Geometry check sheet. Reference: the model listing, model coordinates, mm. Face numbers are marked on the shaded views. A direction names the side the tool comes from. Coordinates: 2 decimals unless noted, no trailing zeros. Loops run counter-clockwise (first coordinate to the right, second up) from the corner with the lowest first, then second, coordinate; pieces in that order, holes last.
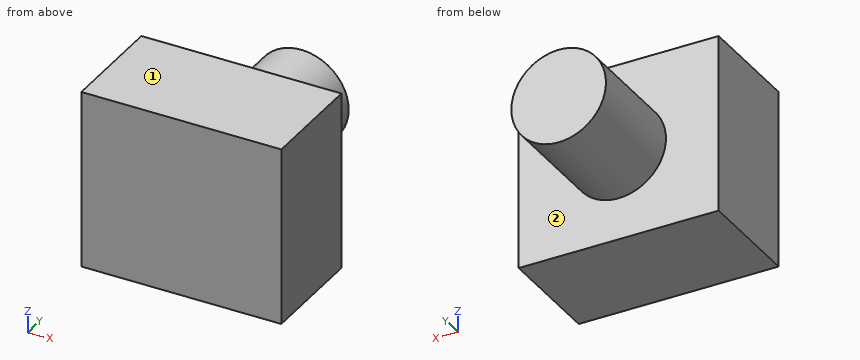
Autodesk Inventor part; units mm, degrees
ref_plane "YZ Plane" through (0, 0, 0) normal (1, 0, 0) x (0, 1, 0)
ref_plane "XZ Plane" through (0, 0, 0) normal (0, 1, 0) x (-1, 0, 0)
ref_plane "XY Plane" through (0, 0, 0) normal (0, 0, 1) x (1, 0, 0)
sketch "Эскиз1" plane through (0, 0, 0) normal (0, 1, 0) x (-1, 0, 0)
  line L0 (3.7, 3.3) -> (-3.7, 3.3)
  line L1 (-3.7, 3.3) -> (-3.7, -3.3)
  line L2 (-3.7, -3.3) -> (3.7, -3.3)
  line L3 (3.7, -3.3) -> (3.7, 3.3)
  point P0 (0, 0)
  dimension "d1" = 6.6
  dimension "d2" = 7.4
  dimension "d3" = 3.3
  dimension "d4" = 3.7
extrude "Выдавливание1" add sketch "Эскиз1" along normal blind 4
sketch "Эскиз2" plane through (0, 4, 0) normal (0, 1, 0) x (1, 0, 0)
  circle A0 centre (0, 0) radius 1.75
  dimension "d7" = 3.5
extrude "Выдавливание2" add sketch "Эскиз2" along normal blind 4
properties part number "btn"
(1) Sectioned sample at C-C on y = 5. Record the cut outline in (x, z), and give its area (3 significant figures).
Findings:
outline: circle Ø3.5 at (0, 0)
area: 9.62 mm2
(2) Access from +Z, -Z, +X, -X, +Y, -Y to the whole of each face (thin tool, end or side, straight path). Record for the marked faces 1 and 2.
Findings:
face 1: +Z, +X, -X, +Y, -Y
face 2: +Y
(3) Sectioned sample at A-A on x = 0. Record the cut outline in (y, z).
Findings:
outline: (0, -3.3) - (4, -3.3) - (4, -1.75) - (8, -1.75) - (8, 1.75) - (4, 1.75) - (4, 3.3) - (0, 3.3) - close
(4) Sectioned sample at D-D on z = -2. Record the cut outline in (x, y).
Findings:
outline: (-3.7, 0) - (3.7, 0) - (3.7, 4) - (-3.7, 4) - close
(5) Sectioned sample at B-B on z = 0. Record the cut outline in (x, y).
Findings:
outline: (-3.7, 0) - (3.7, 0) - (3.7, 4) - (1.75, 4) - (1.75, 8) - (-1.75, 8) - (-1.75, 4) - (-3.7, 4) - close
(6) Gauge pin test, flat ends, axial feed: pin 1 Ø1.5 at (y, z) = (5.5, 0) entering from +X; pin 2 Ø4 at (x, y) = (-2, 7) entering from -Z. Record the tip position at first contact, or that the pin passes through.
Findings:
pin 1: stops at x = 1.75
pin 2: stops at z = -1.75
(7) Scan lines: L1, parallel to Y at x = -2.25, z = -3; L2, parallel to X at y = 7.25, z = -0.75; L3, parallel to X at y = 4.5, z = 0.5. Record each from-to range of solid material in increasing order.
Findings:
L1: y = 0 to 4
L2: x = -1.58 to 1.58
L3: x = -1.68 to 1.68
